Could you check a few things on this model? Use its own coordinates, in mm. Face numbers are marked on the shaded views. A direction names the side the tool comes from. Round coordinates to 2 decimals unless told otherwise and drop trailing zeros. Write each loop counter-clockwise with the first axis right and the second up, starting at its lowest first coordinate (ties: lowest second). Pieces come first, ordered by that corner, then holes. Notation, with made-up numbers: (-28, 80.25) - (0, 80.25) arc R18 cw to (0, 111.25) - close; hole circle Ø6 at (26, -25). An arc over 180 degrees is marked (long way). Write each question's results on one line, items separated by ' | '. Start each with the question number.
(1) On a 3-axis mill with a long thin cutter (end or side, diameter ignored), from which of +Z, -Z, +X, -X, +Y, -Y can I reach the whole of each face in a straight line? I mean the marked faces 4 and 5. Say none if no direction works.
(2) Please list where these lines run through material, in increasing order: line 1 (Y direction, x = 0, z = 0.3); line 2 (Z direction, x = -8, y = 4); line 3 (Z direction, x = -11.5, y = 4.5). Write a range as [from, to].
(3) Thinking about a two-plate mould opening in X: for the marked faces 1, 2 and 3, which applies, +X half, -X half, draft (parallel to the pull), parting line (faces both ways), or undercut?
(4) Imagine slicing it at D-D on z = 21.5. Write out the boundary of the cut face in (x, y), then the cut area to 3 significant figures.
(5) For P1, Ø6, axis at y = 2, z = 31.5, coming from the +X side; P2, Ø8, axis at y = -5, z = 7, coming from the -X side; P3, Ø5, axis at x = 3.5, y = -1, coming from the -Z side, each with a flat end and sliding along its axis, tell me the tip position at first contact or that it passes through.
(6) Imagine slicing it at C-C on z = 46.5. Write out the boundary of the cut face in (x, y), then the cut area to 3 significant figures.
(7) Imagine slicing it at A-A on x = 0. Write out the boundary of the cut face in (y, z), then the cut area to 3 significant figures.
```python
from build123d import *

# Parameters (mm, degrees)
F0_R     = 10
F1_DEPTH = 12
F2_R     = 10
F3_DEPTH = 13
F4_R     = 3.75
F5_DEPTH = 25
F6_R     = 1
F7_R     = 1
F8_DEPTH = 1


with BuildPart() as f1:
    # F0 (on Top) → F1 (new body)
    with BuildSketch(Plane.XY):
        with BuildLine():
            ThreePointArc((-2, 21.4067746286), (-7.8493163593, 7.8493163593), (-21.4067746286, 2))
            ThreePointArc((-21.4067746286, 2), (-21.5, 0), (-21.4067746286, -2))
            ThreePointArc((-21.4067746286, -2), (-7.8493163593, -7.8493163593), (-2, -21.4067746286))
            ThreePointArc((-2, -21.4067746286), (0, -21.5), (2, -21.4067746286))
            ThreePointArc((2, -21.4067746286), (7.8493163593, -7.8493163593), (21.4067746286, -2))
            ThreePointArc((21.4067746286, -2), (21.5, 0), (21.4067746286, 2))
            ThreePointArc((21.4067746286, 2), (7.8493163593, 7.8493163593), (2, 21.4067746286))
            ThreePointArc((2, 21.4067746286), (0, 21.5), (-2, 21.4067746286))
        make_face()
        Circle(F0_R, mode=Mode.SUBTRACT)
        Circle(F0_R)
    extrude(amount=F1_DEPTH)

    # F2 (on face) → F3 (join)
    with BuildSketch(Plane.XY.offset(12)):
        Circle(F2_R)
    extrude(amount=F3_DEPTH)

    # F4 (on face) → F5 (join)
    with BuildSketch(Plane.XY.offset(25)):
        Circle(F4_R)
    extrude(amount=F5_DEPTH)

    # F6
    f6_edges = [f1.edges().sort_by_distance(p)[0] for p in [
        (-10, 0, 25),
    ]]
    fillet(f6_edges, radius=F6_R)

    # F7
    f7_edges = [f1.edges().sort_by_distance(p)[0] for p in [
        (-2, -21.406775, 6),
        (2, -21.406775, 6),
        (-21.406775, -2, 6),
        (-21.406775, 2, 6),
        (-2, 21.406775, 6),
        (2, 21.406775, 6),
        (21.406775, 2, 6),
        (21.406775, -2, 6),
    ]]
    fillet(f7_edges, radius=F7_R)

    # F0 (on Top) → F8 (cut)
    with BuildSketch(Plane.XY):
        Circle(F0_R)
    extrude(amount=F8_DEPTH, mode=Mode.SUBTRACT)


solid = f1.part
```
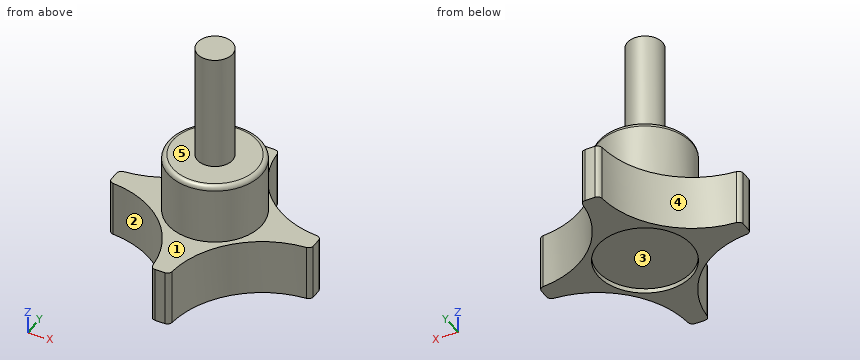
Response:
1) face 4: +Z, -Z, -X, +Y | face 5: +Z
2) line 1: [-21.5, -10], [10, 21.5] | line 2: [1, 25] | line 3: [0, 12]
3) face 1: draft | face 2: -X half | face 3: undercut
4) outline: circle Ø20 at (0, 0) | area: 314 mm²
5) P1: x = 3.75 | P2: x = -21.48 | P3: z = 1
6) outline: circle Ø7.5 at (0, 0) | area: 44.2 mm²
7) outline: (-21.5, 0) - (-10, 0) - (-10, 1) - (10, 1) - (10, 0) - (21.5, 0) - (21.5, 12) - (10, 12) - (10, 24) arc R1 ccw to (9, 25) - (3.75, 25) - (3.75, 50) - (-3.75, 50) - (-3.75, 25) - (-9, 25) arc R1 ccw to (-10, 24) - (-10, 12) - (-21.5, 12) - close | area: 943 mm²
